Part model, mm, in its own coordinate system. A direction names the side the tool comes from. Give positions to 0.01 mm unless a question says otherwise; leave off trailing zeros. Order: outer loops, then holes, each group sorted by start corner. A loop starts at its lowest first (then second) coordinate and runs counter-clockwise, first axis right, second up. Notation, with made-up numbers: M 15,2.25 L 55,2.25 A21 cw 55,41.25 Z; hole C -35,33.5 d1. An arc over 180 degrees is marked long. One line per question, with ' | ' between items.
```python
from build123d import *

# Parameters (mm, degrees)
F2_DEPTH = 5
F3_R     = 2.49999
F4_W     = 80
F4_H     = 32
F5_DEPTH = 0.5
F7_DEPTH = 7
F8_DEPTH = 0.6
F9_R     = 3.49999
F10_R    = 5


# Not quite as in the source:
# - a fillet or chamfer is up to 0.001 mm smaller than in the source, because OpenCascade refuses the exact size


with BuildPart() as f2:
    # F1 (on Front) → F2 (new body)
    with BuildSketch(Plane.XZ):
        Polygon((-40, 32), (-40, 0), (-35, 0), (-35, 27), (35, 27), (35, 0), (40, 0), (40, 32), align=None)
    extrude(amount=F2_DEPTH)

    # F3 (radius 2.5 in the source; OpenCascade refuses exactly that, so slightly less here)
    f3_edges = [f2.edges().sort_by_distance(p)[0] for p in [
        (-35, -5, 13.5),
        (-35, 0, 13.5),
        (40, -5, 16),
        (40, 0, 16),
        (35, -5, 13.5),
        (35, 0, 13.5),
        (0, 0, 27),
        (0, 0, 32),
        (-40, 0, 16),
        (0, -5, 32),
        (-40, -5, 16),
        (0, -5, 27),
    ]]
    fillet(f3_edges, radius=F3_R)

    # F4 (on Front) → F5 (cut)
    with BuildSketch(Plane.XZ):
        with Locations((0, 16)):
            Rectangle(F4_W, F4_H)
    extrude(amount=F5_DEPTH, mode=Mode.SUBTRACT)

    # F6 (on face) → F7 (join)
    with BuildSketch(Plane(origin=(0, -0.5, 0), x_dir=(-1, 0, 0), z_dir=(0, 1, 0))):
        Polygon((-35.9999933333, 0), (-37.5, 0), (-39.0000066667, 0), (-41, 0), (-41, -0.936), (-34, -0.936), (-34, 0), align=None)
        Polygon((41, 0), (39.0000066667, 0), (37.5, 0), (35.9999933333, 0), (34, 0), (34, -0.936), (41, -0.936), align=None)
    extrude(amount=-F7_DEPTH)

    # F6 (on face) → F8 (join)
    with BuildSketch(Plane(origin=(0, -0.5, 0), x_dir=(-1, 0, 0), z_dir=(0, 1, 0))):
        Polygon((-34, -0.936), (-41, -0.936), (-41, -10.936), (0, -10.936), (41, -10.936), (41, -0.936), (34, -0.936), (0, -0.936), align=None)
    extrude(amount=-F8_DEPTH)

    # F9 (radius 3.5 in the source; OpenCascade refuses exactly that, so slightly less here)
    f9_edges = [f2.edges().sort_by_distance(p)[0] for p in [
        (41, -7.5, -0.468),
        (34, -7.5, -0.468),
        (-34, -7.5, -0.468),
        (-41, -7.5, -0.468),
    ]]
    fillet(f9_edges, radius=F9_R)

    # F10
    f10_edges = [f2.edges().sort_by_distance(p)[0] for p in [
        (41, -0.8, -10.936),
        (-41, -0.8, -10.936),
    ]]
    fillet(f10_edges, radius=F10_R)


solid = f2.part
```
1. Slice it at C-C on y = -6.75. Give the cut face in (x, z), then the cut area to 3 significant figures.
Worked out:
outline: M -39.67,-0.94 L -35.33,-0.94 L -35.33,0 L -39.67,0 Z; M 35.33,-0.94 L 39.67,-0.94 L 39.67,0 L 35.33,0 Z | area: 8.11 mm2
2. Drop flat-ended pins along their axis: pin 1 (6 mm diameter, centred on x = -24.5, z = 25.5, fed in from -Y); pin 2 (1.9 mm diameter, centred on x = -38, y = -4.5, fed in from -Z); pin 3 (3 mm diameter, centred on y = -5, z = 3, fed in from -X). Give the stop position or say it passes through.
Worked out:
pin 1: stops at y = -4.79 | pin 2: stops at z = -0.94 | pin 3: stops at x = -39.79
3. Slice it at D-D on y = -3.25. Give the cut face in (x, z), then the cut area to 3 significant figures.
Worked out:
outline: M -41,-0.94 L -34,-0.94 L -34,0 L -35.12,0 L -35.12,27.12 L 35.12,27.12 L 35.12,0 L 34,0 L 34,-0.94 L 41,-0.94 L 41,0 L 39.88,0 L 39.88,31.88 L -39.88,31.88 L -39.88,0 L -41,0 Z | area: 652 mm2
4. Probe L1, parallel to X at y = -4.5, z = 23; L2, parallel to X at y = -2.25, z = 17; L3, parallel to Y at x = -37, z = -6.5. List the from-to ranges inside material, lowest first. Write a range as from..to.
Worked out:
L1: x = -39..-36, 36..39 | L2: x = -39.99..-35.01, 35.01..39.99 | L3: y = -1.1..-0.5
5. Mould opens along X. For faces 1 (the cylindrical face through (35.257, -1.396, 13.804)), 2 (the flat face through (1, -1.1, -6)), 3 (the cylindrical face through (39.574, -0.804, -9.432)) say: released by +X, released by -X, zero draft, split by the parting line, or undercut.
Worked out:
face 1: undercut | face 2: zero draft | face 3: released by +X
6. Tool access for faces 4 (the cylindrical face through (-39.287, -4.248, 15.776)), 5 (the cylindrical face through (0.504, -1.396, 27.257)), 6 (the cylindrical face through (-35, -6.45, -0.47)), 7 (the cylindrical face through (35.713, -4.248, 14.543)), 8 (the flat face through (-37, -4, -0.936)): list every direction of +Z, -Z, +X, -X, +Y, -Y with a clear straight run to the whole face (end or side of a thin tool).
Worked out:
face 4: +Z, -X, -Y | face 5: +Y | face 6: -Z, -Y | face 7: -Y | face 8: -Z, +X, -X, -Y
